Print and shaded views of the part. All mm, measured from the part's lowest x, y and z. Coordinates: 2 decimals unless noted, no trailing zeros. Order: outer loops, then holes, each group sorted by start corner. A loop starts at its lowest first (then second) coordinate and runs counter-clockwise, first axis right, second up. Notation, with made-up numbers: M 45.25,56 L 96.25,56 A12 ccw 96.25,73 Z; hole C -14.5,35 d11. An arc over 180 degrees is marked long. Return JSON: item names as keys, results as strings.
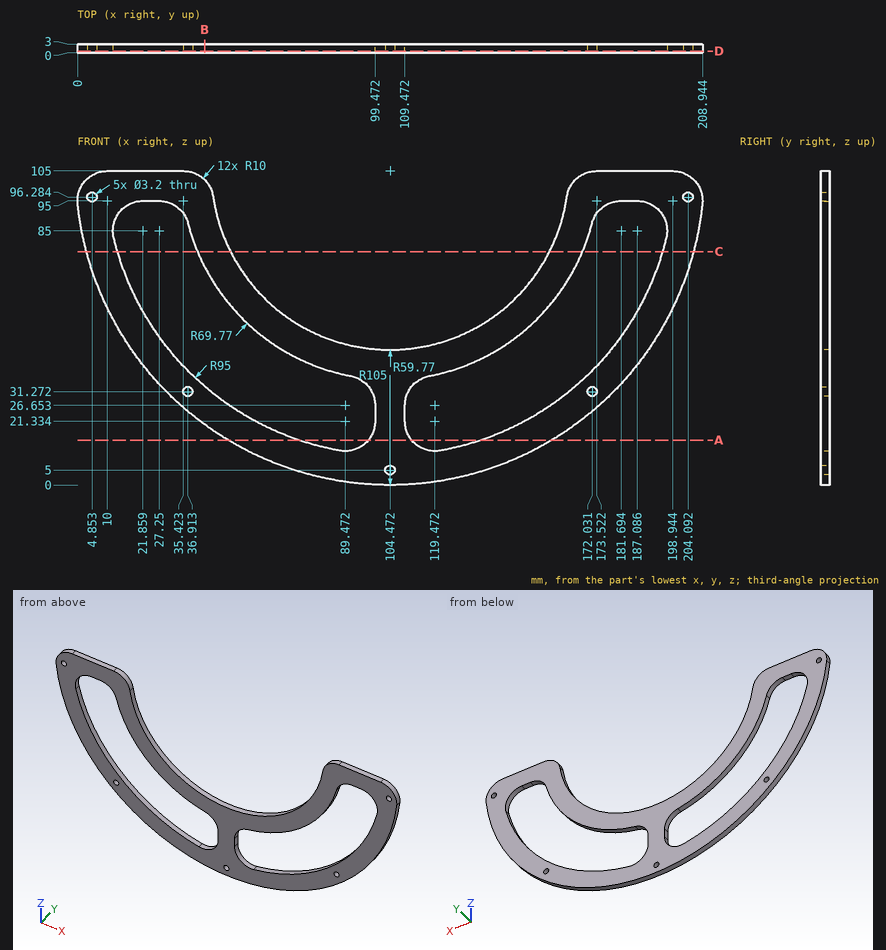
Item 1: Saw through at C-C (z = 78). Write the cut outline in (x, y) (1 decimal).
Check result:
{"outline": "M 3,0 L 13.4,0 L 13.4,3 L 3,3 Z; M 40.1,0 L 51.1,0 L 51.1,3 L 40.1,3 Z; M 157.8,0 L 168.8,0 L 168.8,3 L 157.8,3 Z; M 195.6,0 L 205.9,0 L 205.9,3 L 195.6,3 Z"}
Item 2: Saw through at B-B (x = 42.5). Write the cut outline in (y, z) (1 decimal).
Check result:
{"outline": "M 0,20.2 L 3,20.2 L 3,33 L 0,33 Z; M 0,72.9 L 3,72.9 L 3,102.1 L 0,102.1 Z"}
Item 3: Saw through at D-D (y = 0.6). Count the separate pieces of the cut face and the enclosed holes in it, and give its area (3 significant figures).
Check result:
{"separate pieces": "1", "enclosed holes": "7", "area": "5,990 mm2"}
Item 4: Drop flat-ended pins along their axis: pin 1 Ø1.5 at (y, z) = (2, 24.5) entering from -X; pin 2 Ø0.9 at (y, z) = (1.5, 24) entering from +X; pin 3 Ø1.9 at (x, z) = (104.47, 5) entering from -Y; pin 4 Ø0.9 at (x, y) = (24.5, 1.5) entering from -Z (1 decimal). Give the stop position or say it passes through.
Check result:
{"pin 1": "stops at x = 36.17", "pin 2": "stops at x = 171.83", "pin 3": "passes through", "pin 4": "stops at z = 36.4"}
Item 5: Wall check: line 1 (X direction, y = 2.3, z = 73) (1 decimal); line 2 (Z direction, x = 173, y = 1.1) (1 decimal); line 3 (X direction, y = 2.3, z = 71) (1 decimal). Give the ranges that are in metal, low to high.
Check result:
{"line 1": "x = 4.5 to 15, 42.5 to 54, 155 to 166.5, 193.9 to 204.5", "line 2": "z = 25.4 to 30, 32.5 to 39.2, 89.9 to 105", "line 3": "x = 5.1 to 15.8, 43.5 to 55.3, 153.6 to 165.4, 193.2 to 203.8"}
Item 6: Saw through at A-A (z = 15). Write the cut outline in (x, y) (1 decimal).
Check result:
{"outline": "M 50.4,0 L 74.1,0 L 74.1,3 L 50.4,3 Z; M 97.2,0 L 111.7,0 L 111.7,3 L 97.2,3 Z; M 134.9,0 L 158.6,0 L 158.6,3 L 134.9,3 Z"}
